from build123d import *

# Parameters (mm, degrees)
F0_W     = 30
F0_H     = 5
F1_DEPTH = 8
F2_R     = 4.25
F3_DEPTH = 5
F4_R     = 5.2
F5_DEPTH = 1.7
F6_R     = 1.5
F7_DEPTH = 8.001


with BuildPart() as f1:
    # F0 (on Top) → F1 (new body)
    with BuildSketch(Plane.XY):
        Rectangle(F0_W, F0_H)
    extrude(amount=F1_DEPTH)

    # F2 (on Front) → F3 (cut, symmetric)
    with BuildSketch(Plane.XZ):
        Circle(F2_R)
    extrude(amount=F3_DEPTH, both=True, mode=Mode.SUBTRACT)

    # F4 (on Front) → F5 (cut, symmetric)
    with BuildSketch(Plane.XZ):
        Circle(F4_R)
    extrude(amount=F5_DEPTH, both=True, mode=Mode.SUBTRACT)

    # F6 (on face) → F7 (cut, through all)
    with BuildSketch(Plane.XY.offset(8)):
        with Locations((-10, 0)):
            Circle(F6_R)
        with Locations((10, 0)):
            Circle(F6_R)
    extrude(amount=-F7_DEPTH, mode=Mode.SUBTRACT)


solid = f1.part
Verification items for the finished model (mm, model axes). A direction names the side the tool comes from. Coordinates: 2 decimals unless noted, no trailing zeros. Write each loop counter-clockwise with the first axis right and the second up, starting at its lowest first coordinate (ties: lowest second). Pieces come first, ordered by that corner, then holes. Notation, with made-up numbers: M 25,50.25 L 51,50.25 A30 cw 51,77.25 Z; hole C -38.5,52.5 d8. An arc over 180 degrees is marked long. Use a Markdown table: item, result.
Q1. Sectioned sample at A-A, the plane y = 0. Record the boundary of the cut face in (x, z).
Reply:
| item | result |
|---|---|
| outline | M -15,0 L -11.5,0 L -11.5,8 L -15,8 Z; M -8.5,0 L -5.2,0 A5.2 cw 5.2,0 L 8.5,0 L 8.5,8 L -8.5,8 Z; M 11.5,0 L 15,0 L 15,8 L 11.5,8 Z |
Q2. Thickness scan on line 1 (Y direction, x = 10, z = 3.75); line 2 (X direction, y = 1.35, z = 5.5); line 3 (X direction, y = -0.45, z = 7.75). Record the ranges inside material, lowest first.
Reply:
| item | result |
|---|---|
| line 1 | y = -2.5 to -1.5, 1.5 to 2.5 |
| line 2 | x = -15 to -10.65, -9.35 to 9.35, 10.65 to 15 |
| line 3 | x = -15 to -11.43, -8.57 to 8.57, 11.43 to 15 |
Q3. Set-up check for faces 4 (the face through (-0.79, -1.7, 4.35)), 5 (the face through (-10, 2, 0)): record each of +Z, -Z, +X, -X, +Y, -Y from which the full face is reachable in a straight line by a thin tool's end or side.
Reply:
| item | result |
|---|---|
| face 4 | -Z |
| face 5 | -Z, +X, -X, +Y, -Y |
Q4. Go/stop test with a flat-tipped pin: P1, Ø2.5, axis at x = -10, y = 0, coming from the +Z side. Record where the tip stops, or that it passes through.
Reply:
| item | result |
|---|---|
| P1 | passes through |
Q5. Sectioned sample at B-B, the plane x = -10. Record the boundary of the cut face in (y, z), plus the area to 3 significant figures.
Reply:
| item | result |
|---|---|
| outline | M -2.5,0 L -1.5,0 L -1.5,8 L -2.5,8 Z; M 1.5,0 L 2.5,0 L 2.5,8 L 1.5,8 Z |
| area | 16.0 mm² |
Q6. Draft check along X on faces 1 (the face through (-0.79, 1.7, 4.35)), 2 (the face through (-15, 0, 4)), 3 (the face through (0, -2.5, 5)). Enter one of: +X half, -X half, draft (parallel to the pull), parting line (faces both ways), or undercut.
Reply:
| item | result |
|---|---|
| face 1 | undercut |
| face 2 | -X half |
| face 3 | draft |
Q7. Sectioned sample at D-D, the plane x = 0. Record the boundary of the cut face in (y, z).
Reply:
| item | result |
|---|---|
| outline | M -2.5,4.25 L -1.7,4.25 L -1.7,5.2 L 1.7,5.2 L 1.7,4.25 L 2.5,4.25 L 2.5,8 L -2.5,8 Z |
Q8. Sectioned sample at C-C, the plane z = 1.25. Record the boundary of the cut face in (x, y), plus the area to 3 significant figures.
Reply:
| item | result |
|---|---|
| outline | M -15,-2.5 L -4.06,-2.5 L -4.06,-1.7 L -5.05,-1.7 L -5.05,1.7 L -4.06,1.7 L -4.06,2.5 L -15,2.5 Z; M 4.06,-2.5 L 15,-2.5 L 15,2.5 L 4.06,2.5 L 4.06,1.7 L 5.05,1.7 L 5.05,-1.7 L 4.06,-1.7 Z; hole C -10,0 d3; hole C 10,0 d3 |
| area | 88.5 mm² |
